Check sheet for the modelled part. Datum: model origin and axes. Units: mm. Face numbers are marked on the shaded views. A direction names the side the tool comes from. Round coordinates to 2 decimals unless told otherwise and drop trailing zeros. Write each loop counter-clockwise with the first axis right and the second up, starting at its lowest first coordinate (ties: lowest second). Pieces come first, ordered by that corner, then holes. Notation, with made-up numbers: (8, 34.25) -> (36, 34.25) arc R27 cw to (36, 63.25) -> close; hole circle Ø10 at (36.25, -27). An arc over 180 degrees is marked (long way). Answer as a JSON object with one key per item and string values. Group by question number.
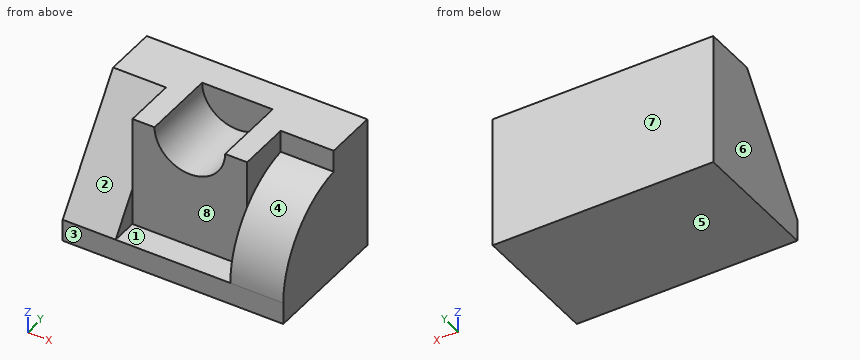
```python
from build123d import *

# Parameters (mm, degrees)
F0_W     = 30
F0_H     = 30
F1_DEPTH = 50
F3_DEPTH = 12
F5_DEPTH = 12
F7_DEPTH = 6
F8_DEPTH = 23


with BuildPart() as f1:
    # F0 (on Right) → F1 (new body)
    with BuildSketch(Plane.YZ):
        with Locations((15, 15)):
            Rectangle(F0_W, F0_H)
    extrude(amount=F1_DEPTH)

    # F2 (on face) → F3 (cut)
    with BuildSketch(Plane.YZ.offset(50)):
        with BuildLine():
            Line((18, 25), (18, 30))
            Line((18, 30), (0, 30))
            Line((0, 30), (0, 5))
            ThreePointArc((0, 5), (5.16264, 18.453624), (18, 25))
        make_face()
    extrude(amount=-F3_DEPTH, mode=Mode.SUBTRACT)

    # F4 (on face) → F5 (cut)
    with BuildSketch(Plane(origin=(0, 0, 0), x_dir=(0, -1, 0), z_dir=(-1, 0, 0))):
        Polygon((0, 30), (-18, 30), (0, 5), align=None)
    extrude(amount=-F5_DEPTH, mode=Mode.SUBTRACT)

    # F6 (on face) → F7 (cut)
    with BuildSketch(Plane.XZ):
        with BuildLine():
            Line((12, 30), (12, 5))
            Line((12, 5), (38, 5))
            Line((38, 5), (38, 30))
            Line((38, 30), (33, 30))
            ThreePointArc((33, 30), (25, 22), (17, 30))
            Line((17, 30), (12, 30))
        make_face()
        with BuildLine():
            Line((33, 30), (17, 30))
            ThreePointArc((17, 30), (25, 22), (33, 30))
        make_face()
    extrude(amount=-F7_DEPTH, mode=Mode.SUBTRACT)

    # F6 (on face) → F8 (cut)
    with BuildSketch(Plane.XZ):
        with BuildLine():
            Line((33, 30), (17, 30))
            ThreePointArc((17, 30), (25, 22), (33, 30))
        make_face()
    extrude(amount=-F8_DEPTH, mode=Mode.SUBTRACT)


solid = f1.part
```
(1) Access from +Z, -Z, +X, -X, +Y, -Y to the whole of each face (thin tool, end or side, straight path). Record for the marked faces 1, 2, 3, 4 and 5.
(2) Section check D-D on x = 8. Record the cut outline in (y, z), then the cut area to 3 significant figures.
(3) Section check C-C on y = 13. Record the cut outline in (x, z), then the cut area to 3 significant figures.
(4) Section check A-A on x = 25. Record the cut outline in (y, z), then the cut area to 3 significant figures.
(5) Section check B-B on z = 17. Record the cut outline in (x, y).
(6) Release check for a two-part mould opening along X. For the marked faces 6, 7 and 8 record: pulls with the +X half, pulls with the -X half, needs draft (parallel to the pull), parting line crosses it, or undercut.
(7) Go/stop test with flat-tipped pins: pin 1 Ø3.5 at (y, z) = (11.5, 25) entering from -X; pin 2 Ø6.5 at (x, y) = (20.5, 1.5) entering from +Z; pin 3 Ø4 at (x, z) = (45, 27.5) entering from -Y. Record where each tip stops, or that it passes through.
(8) Scan lines: line 1 along X through (y, z) = (4, 6.75); line 2 along Y through (x, z) = (32, 21.5); line 3 along X through (y, z) = (2.75, 12.25). Record each from-to range of solid material in increasing order.
Data:
{
 "1": {"face 1": "+Z, -Y", "face 2": "+Z, -X, -Y", "face 3": "+Z, -Z, +X, -X, -Y", "face 4": "+Z, +X, -Y", "face 5": "-Z, +X, -X, +Y, -Y"},
 "2": {"outline": "(0, 0) -> (30, 0) -> (30, 30) -> (18, 30) -> (0, 5) -> close", "area": "675 mm²"},
 "3": {"outline": "(0, 0) -> (50, 0) -> (50, 23.81) -> (38, 23.81) -> (38, 30) -> (33, 30) arc R8 cw to (17, 30) -> (12, 30) -> (12, 23.06) -> (0, 23.06) -> close", "area": "1,240 mm²"},
 "4": {"outline": "(0, 0) -> (30, 0) -> (30, 30) -> (23, 30) -> (23, 22) -> (6, 22) -> (6, 5) -> (0, 5) -> close", "area": "614 mm²"},
 "5": {"outline": "(0, 8.64) -> (12, 8.64) -> (12, 6) -> (38, 6) -> (38, 3.97) -> (50, 3.97) -> (50, 30) -> (0, 30) -> close"},
 "6": {"face 6": "pulls with the -X half", "face 7": "needs draft", "face 8": "undercut"},
 "7": {"pin 1": "stops at x = 12", "pin 2": "stops at z = 5", "pin 3": "stops at y = 18"},
 "8": {"line 1": "x = 0 to 12, 38 to 50", "line 2": "y = 6 to 30", "line 3": "x = 38 to 50"}
}
